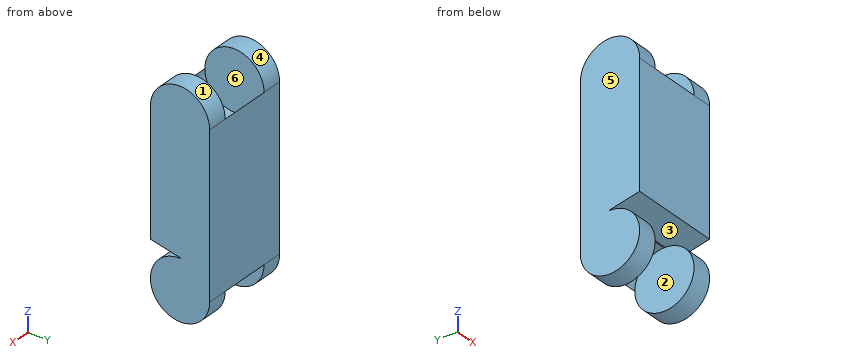
from build123d import *

# Parameters (mm, degrees)
F1_DEPTH = 57.15
F2_START = 31.75
F2_DEPTH = 25.4
F3_START = -31.75
F3_DEPTH = 25.4
F4_START = 31.75
F4_DEPTH = 25.4
F5_START = -31.75
F5_DEPTH = 25.4


with BuildPart() as f1:
    # F0 (on Right) → F1 (new body, symmetric)
    with BuildSketch(Plane.YZ):
        with BuildLine():
            Line((37.1475, -74.295), (37.1475, 0))
            ThreePointArc((37.1475, 0), (0, -37.1475), (-37.1475, 0))
            Line((-37.1475, 0), (-37.1475, -74.295))
            Line((-37.1475, -74.295), (37.1475, -74.295))
        make_face()
        with BuildLine():
            Line((37.1475, -201.295), (37.1475, -74.295))
            Line((37.1475, -74.295), (-37.1475, -74.295))
            Line((-37.1475, -74.295), (-37.1475, -155.7949632406))
            Line((-37.1475, -155.7949632406), (0, -163.3808536928))
            Line((0, -163.3808536928), (0.7587369735, -164.1552494024))
            ThreePointArc((0.7587369735, -164.1552494024), (26.5341472255, -175.2973888162), (37.1475, -201.295))
        make_face()
    extrude(amount=F1_DEPTH, both=True)

    # F0 (on Right) → F2 (join)
    with BuildSketch(Plane.YZ.offset(F2_START)):
        with BuildLine():
            Line((-37.1475, 0), (37.1475, 0))
            ThreePointArc((37.1475, 0), (0, 37.1475), (-37.1475, 0))
        make_face()
        with BuildLine():
            ThreePointArc((-37.1475, 0), (0, -37.1475), (37.1475, 0))
            Line((37.1475, 0), (-37.1475, 0))
        make_face()
    extrude(amount=F2_DEPTH)

    # F0 (on Right) → F3 (join)
    with BuildSketch(Plane.YZ.offset(F3_START)):
        with BuildLine():
            Line((-37.1475, 0), (37.1475, 0))
            ThreePointArc((37.1475, 0), (0, 37.1475), (-37.1475, 0))
        make_face()
        with BuildLine():
            ThreePointArc((-37.1475, 0), (0, -37.1475), (37.1475, 0))
            Line((37.1475, 0), (-37.1475, 0))
        make_face()
    extrude(amount=-F3_DEPTH)

    # F0 (on Right) → F4 (join)
    with BuildSketch(Plane.YZ.offset(F4_START)):
        with BuildLine():
            Line((-37.1475, -201.295), (37.1475, -201.295))
            Line((37.1475, -201.295), (0.7587369735, -164.1552494024))
            ThreePointArc((0.7587369735, -164.1552494024), (-25.9976111838, -174.7608527745), (-37.1475, -201.295))
        make_face()
        with BuildLine():
            ThreePointArc((-37.1475, -201.295), (0, -238.4425), (37.1475, -201.295))
            Line((37.1475, -201.295), (-37.1475, -201.295))
        make_face()
        with BuildLine():
            Line((0.7587369735, -164.1552494024), (37.1475, -201.295))
            ThreePointArc((37.1475, -201.295), (26.5341472255, -175.2973888162), (0.7587369735, -164.1552494024))
        make_face()
    extrude(amount=F4_DEPTH)

    # F0 (on Right) → F5 (join)
    with BuildSketch(Plane.YZ.offset(F5_START)):
        with BuildLine():
            Line((-37.1475, -201.295), (37.1475, -201.295))
            Line((37.1475, -201.295), (0.7587369735, -164.1552494024))
            ThreePointArc((0.7587369735, -164.1552494024), (-25.9976111838, -174.7608527745), (-37.1475, -201.295))
        make_face()
        with BuildLine():
            ThreePointArc((-37.1475, -201.295), (0, -238.4425), (37.1475, -201.295))
            Line((37.1475, -201.295), (-37.1475, -201.295))
        make_face()
        with BuildLine():
            Line((0.7587369735, -164.1552494024), (37.1475, -201.295))
            ThreePointArc((37.1475, -201.295), (26.5341472255, -175.2973888162), (0.7587369735, -164.1552494024))
        make_face()
    extrude(amount=-F5_DEPTH)


solid = f1.part
Build history of the part. All positions in model axes, mm. Face numbers are marked on the shaded views. A direction names the side the tool comes from. Round coordinates to 2 decimals unless told otherwise and drop trailing zeros. Loops run counter-clockwise (first coordinate to the right, second up) from the corner with the lowest first, then second, coordinate; pieces in that order, holes last. Notation, with made-up numbers: (-40, 72) -> (-8, 72) arc R18 cw to (-8, 99) -> close; hole circle Ø5 at (-5, 73.25). An arc over 180 degrees is marked (long way). Use CSV: the item, a comma, the result in double quotes. Start each with the question number.
Q1. Saw through at B-B on x = 26.5. Give the cut face in (y, z) (1 decimal).
Q2. Drill centre lines: L1, parallel to X at y = -11, z = -7.5; L2, parallel to Z at x = 36, y = -20; L3, parallel to Z at x = -32.5, y = -15. Where is each one in solid material? Low to high.
Q3. Mould opens along Y. For the marked faces 3, 4, 5 and 6 say: +Y half, -Y half, draft (parallel to the pull), parting line (faces both ways), or undercut.
Q4. Saw through at A-A on y = -22.5. Give the cut face in (x, z), and give its area (3 significant figures).
Q5. Saw through at C-C on y = 29.5. Give the cut face in (x, z), and give its area (3 significant figures).
Q6. Saw through at D-D on x = 47. Give the cut face in (y, z) (1 decimal).
Q7. Flat gauge pins, fed straight in: pin 1 Ø8 at (x, y) = (27, 21.5) entering from +Z; pin 2 Ø8 at (x, y) = (-1.5, 24.5) entering from -Z; pin 3 Ø1 at (x, y) = (-41.5, 20.5) entering from -Z. Where does each tip first touch, or does it go through?
Q8. Which spindle directions (+Z, -Z, +X, -X, +Y, -Y) get a long thin tool onto all of the face, cutting with end or side? Do the marked faces 1 and 2. Say none if no direction does.
Solutions:
1,outline,"(-37.1, -155.8) -> (0, -163.4) -> (0.8, -164.2) arc R37.1 cw to (37.1, -201.3) -> (37.1, 0) arc R37.1 cw to (-37.1, 0) -> close"
2,L1,"x = -57.15 to -31.75, 31.75 to 57.15"
2,L2,"z = -232.6 to -169.99, -159.3 to 31.3"
2,L3,"z = -235.28 to -167.31, -160.32 to 33.98"
3,face 3,"-Y half"
3,face 4,"parting line"
3,face 5,"draft"
3,face 6,"undercut"
4,outline,"(-57.15, -230.85) -> (-31.75, -230.85) -> (-31.75, -171.74) -> (-57.15, -171.74) -> close; (-57.15, -158.79) -> (57.15, -158.79) -> (57.15, 29.56) -> (31.75, 29.56) -> (31.75, -29.56) -> (-31.75, -29.56) -> (-31.75, 29.56) -> (-57.15, 29.56) -> close; (31.75, -230.85) -> (57.15, -230.85) -> (57.15, -171.74) -> (31.75, -171.74) -> close"
4,area,"20,800 mm^2"
5,outline,"(-57.15, -223.87) -> (-31.75, -223.87) -> (-31.75, -178.72) -> (31.75, -178.72) -> (31.75, -223.87) -> (57.15, -223.87) -> (57.15, 22.58) -> (31.75, 22.58) -> (31.75, -22.58) -> (-31.75, -22.58) -> (-31.75, 22.58) -> (-57.15, 22.58) -> close"
5,area,"22,400 mm^2"
6,outline,"(-37.1, -155.8) -> (0, -163.4) -> (0.8, -164.2) arc R37.1 ccw (long way) to (37.1, -201.3) -> (37.1, 0) arc R37.1 ccw to (-37.1, 0) -> close"
7,pin 1,"stops at z = -27.01"
7,pin 2,"stops at z = -177.47"
7,pin 3,"stops at z = -232.6"
8,face 1,"+Z, +X, -X"
8,face 2,"-Z, -Y"
